Design review of the part built by this model. Coordinates are the model's own, in mm. Round coordinates to 2 decimals unless told otherwise and drop trailing zeros. Order: outer loops, then holes, each group sorted by start corner. A loop starts at its lowest first (then second) coordinate and runs counter-clockwise, first axis right, second up. Notation, with made-up numbers: (79, 47.5) - (117, 47.5) arc R32 cw to (117, 73.5) - close; hole circle Ø5 at (-7, -29). An arc over 180 degrees is marked (long way). Use CSV: the item, a comma, the result in double quotes.
from build123d import *

# Parameters (mm, degrees)
SKETCH1_R           = 292.5
SKETCH1_R_2         = 45
BOSS_EXTRUDE1_DEPTH = 4
SKETCH2_R           = 4.5
CUT_EXTRUDE1_DEPTH  = 414.676806215
CIRPATTERN1_COUNT   = 12
CIRPATTERN3_COUNT   = 3


with BuildPart() as part:
    # Sketch1 → Boss-Extrude1 (new body)
    with BuildSketch(Plane.XY):
        Circle(SKETCH1_R)
        Circle(SKETCH1_R_2, mode=Mode.SUBTRACT)
    extrude(amount=BOSS_EXTRUDE1_DEPTH)

    # Sketch2 → Cut-Extrude1 (cut, through all)
    with BuildSketch(Plane.XY.offset(4)):
        with Locations((0, 275)):
            Circle(SKETCH2_R)
    cut_extrude1 = extrude(amount=-CUT_EXTRUDE1_DEPTH, mode=Mode.SUBTRACT)

    # CirPattern1: Cut-Extrude1 ×12 about axis
    cirpattern1_axis = Axis((0, 0, 0), (0, 0, 1))
    for i in range(1, CIRPATTERN1_COUNT):
        add(cut_extrude1.rotate(cirpattern1_axis, i * 360 / CIRPATTERN1_COUNT), mode=Mode.SUBTRACT)

    # Sketch6 → M6x1.0 Tapped Hole1 (revolve, cut)
    with BuildSketch(Plane(origin=(0, 55, 0), x_dir=(0, 1, 0), z_dir=(1, 0, 0))):
        Polygon((0, 0), (0, 16.502151548), (2.5, 15), (2.5, 0), align=None)
    m6x1_0_tapped_hole1 = revolve(axis=Axis((0, 55, -6.35), (0, 0, 1)), mode=Mode.SUBTRACT)

    # CirPattern3: M6x1.0 Tapped Hole1 ×3 about axis
    cirpattern3_axis = Axis((0, 0, 0), (0, 0, 1))
    for i in range(1, CIRPATTERN3_COUNT):
        add(m6x1_0_tapped_hole1.rotate(cirpattern3_axis, i * 360 / CIRPATTERN3_COUNT), mode=Mode.SUBTRACT)


solid = part.part
1) We need section B-B (x = -35). Give the boundary of the cut face in (y, z).
Data:
outline,"(-290.4, 0) - (-28.28, 0) - (-28.28, 4) - (-290.4, 4) - close; (28.28, 0) - (290.4, 0) - (290.4, 4) - (28.28, 4) - close"
2) The part is to be moulded in two halves that separate along Y. For faces 1 (the face through (278.993, 87.859, 1.972)), 2 (the face through (20.765, -39.923, 1.972)), 3 (the face through (61, 4, 4)), say which applies: +Y half, -Y half, draft (parallel to the pull), parting line (faces both ways), or undercut.
Data:
face 1,"parting line"
face 2,"undercut"
face 3,"draft"
3) Insertion check: pin 1 Ø2 at (y, z) = (-26.5, 2) entering from -X; pin 2 Ø2 at (y, z) = (-153, 2) entering from -X; pin 3 Ø2 at (y, z) = (-151, 1) entering from -X. Each pin has a flat end and moves straight along its axis. Give the tip position at first contact, or say it passes through.
Data:
pin 1,"stops at x = -291.39"
pin 2,"stops at x = -249.9"
pin 3,"stops at x = -251.11"
4) We need section A-A (z = 3.35). Give the number of separate pieces and of enclosed holes in the cut face, then the cut area to 3 significant figures.
Data:
separate pieces,"1"
enclosed holes,"16"
area,"262,000 mm2"
5) We need section C-C (y = -57). Give the boundary of the cut face in (x, z), then the cut area to 3 significant figures.
Data:
outline,"(-286.89, 0) - (286.89, 0) - (286.89, 4) - (-286.89, 4) - close"
area,"2,300 mm2"
6) We need section D-D (x = 226.5). Give the boundary of the cut face in (y, z).
Data:
outline,"(-185.08, 0) - (185.08, 0) - (185.08, 4) - (-185.08, 4) - close"
7) To check wall thickness, follow L1, parallel to Y at x = 0, z = 1.7; L2, parallel to X at y = -27.5, z = 1.05; L3, parallel to Y at x = -49, z = 1.45. State the ranges of each line that lie inside material, in increasing order. Write a range as from..to.
Data:
L1,"y = -292.5..-279.5, -270.5..-45, 45..52.5, 57.5..270.5, 279.5..292.5"
L2,"x = -291.2..-50.13, -45.13..-35.62, 35.62..45.13, 50.13..291.2"
L3,"y = -288.37..-29.59, -25.41..288.37"
